Can you work these out from the model? Positions are in its coordinate system, mm. Face numbers are marked on the shaded views. Coordinates: 2 decimals unless noted, no trailing zeros. Order: outer loops, then holes, each group sorted by start corner. A loop starts at its lowest first (then second) coordinate and runs counter-clockwise, first axis right, second up.
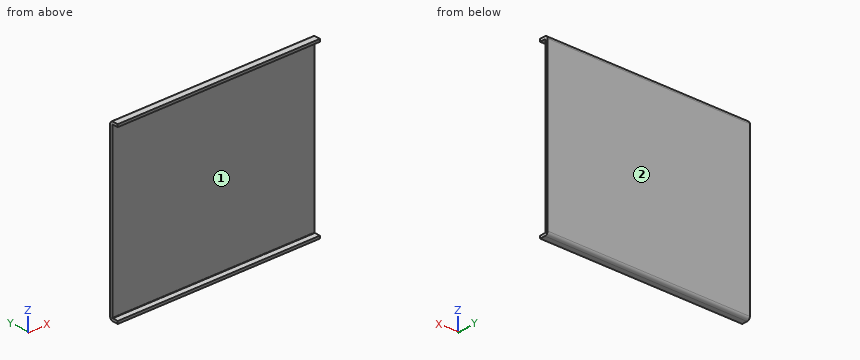
Autodesk Inventor part; units mm, degrees
ref_plane "YZ Plane" through (0, 0, 0) normal (1, 0, 0) x (0, 1, 0)
ref_plane "XZ Plane" through (0, 0, 0) normal (0, 1, 0) x (-1, 0, 0)
ref_plane "XY Plane" through (0, 0, 0) normal (0, 0, 1) x (1, 0, 0)
sketch "Sketch1" plane through (0, 0, 0) normal (0, 1, 0) x (-1, 0, 0)
  line L0 (60, -50) -> (-60, -50)
  line L1 (-60, -50) -> (-60, 50)
  line L2 (-60, 50) -> (60, 50)
  line L3 (60, 50) -> (60, -50)
  point P0 (0, 0)
  dimension "d0" = 120
  dimension "d1" = 100
  dimension "d2" = 50
  dimension "d3" = 60
extrude "Plate1" add sketch "Sketch1" along normal blind 1.5
sketch "Sketch2" plane through (60, 1.5, -48.5) normal (0, 0, -1) x (-1, 0, 0)
  line L0 (120, 0) -> (0, 0)
  line L1 (0, 0) -> (0, -5)
  line L2 (0, -5) -> (120, -5)
  line L3 (120, -5) -> (120, 0)
edge flange "Flange1" height 5 angle 90 thickness 1.5 bend radius 0.31 thickness toward (0, 0, -1) relief tear relief width 1.5 relief depth 0.75 corner gap 0.31 corner form 0 edges at (0, 0, -50) (0, 0, 50) wall of the first edge with corners at (-60, 1.5, -48.5) (60, 1.5, -48.5) (60, -3.5, -48.5) (-60, -3.5, -48.5)
bend "Bend1"
corner "Corner1"
equation "\"d4\" = Thickness"
equation "\"d5\" = BendReliefWidth"
equation "\"d6\" = BendReliefDepth"
equation "\"d7\" = MinimumRemnant"
equation "\"d8\" = TransitionRadius"
equation "\"d11\" = BendRadius"
equation "\"d12\" = CornerReliefSize"
equation "\"d13\" = GapSize"
equation "\"d14\" = JacobiRadiusSize"
equation "\"BendReliefWidth\" = Thickness"
equation "\"BendReliefDepth\" = 0.5 * Thickness"
equation "\"CornerReliefSize\" = 4 * Thickness"
equation "\"MinimumRemnant\" = 2 * Thickness"
equation "\"TransitionRadius\" = BendRadius"
equation "\"JacobiRadiusSize\" = BendRadius"
equation "\"GapSize\" = Thickness"
properties part number "axis_12_bottom_frame(bottom)" material "Aluminum 6061-AHC"
1. Please list where these lines run through material, in increasing order: probe 1 along Z at (x, y) = (42, -2.1); probe 2 along Y at (x, z) = (52, 17); probe 3 along Z at (x, y) = (53, 0.55).
Completed:
probe 1: z = -50 to -48.5, 48.5 to 50
probe 2: y = 0 to 1.5
probe 3: z = -49.78 to 49.78
2. Imagine slicing it at C-C on z = 5. Please give me the cut outline in (x, y).
Completed:
outline: (-60, 0) - (60, 0) - (60, 1.5) - (-60, 1.5) - close
3. Imagine slicing it at B-B on x = 40.5. Please give me the cut outline in (y, z), then the cut area to 3 significant figures.
Completed:
outline: (-3.5, -50) - (-0.31, -50) arc R1.81 ccw to (1.5, -48.19) - (1.5, 48.19) arc R1.81 ccw to (-0.31, 50) - (-3.5, 50) - (-3.5, 48.5) - (-0.31, 48.5) arc R0.31 cw to (0, 48.19) - (0, -48.19) arc R0.31 cw to (-0.31, -48.5) - (-3.5, -48.5) - close
area: 159 mm2
4. Imagine slicing it at A-A on y = -2.1. Please give me the cut outline in (x, z), then the cut area to 3 significant figures.
Completed:
outline: (-60, -50) - (60, -50) - (60, -48.5) - (-60, -48.5) - close; (-60, 48.5) - (60, 48.5) - (60, 50) - (-60, 50) - close
area: 360 mm2
5. Thinking about a two-plate mould opening in Z: for the marked faces 1 and 2, which applies, pulls with the +Z half, pulls with the -Z half, needs draft (parallel to the pull), parting line crosses it, or undercut?
Completed:
face 1: undercut
face 2: needs draft
6. I'm going to push a flat-ended pin straight in: pin 1 (6 mm diameter, centred on x = 36.5, z = -30, fed in from -Y). Where does the tip first touch, or does it pass through?
Completed:
pin 1: stops at y = 0
